```python
from build123d import *

# Parameters (mm, degrees)
F2_R = 5.08


with BuildPart() as f1:
    # F0 (on Right) → F1 (revolve)
    with BuildSketch(Plane.YZ):
        Polygon((-64.897239, 0), (0, 0), (86.770147, 0), (93.20876, 4.190467), (93.20876, 11.651084), (89.325145, 22.790901), (81.864543, 22.790901), (77.878736, 14.819287), (73.484123, 7.767476), (59.891507, 7.767476), (56.518897, 12.67308), (51.000088, 19.827098), (44.970281, 24.630502), (32.7297, 28.463185), (22.135049, 28.463185), (11.288136, 24.301), (4.981786, 17.364018), (0, 9.039648), (-64.897239, 9.039648), align=None)
    revolve(axis=Axis((0, -32.44862, 0), (0, -1, 0)))

    # F2
    f2_edges = [f1.edges().sort_by_distance(p)[0] for p in [
        (0, -64.897239, -9.039648),
    ]]
    fillet(f2_edges, radius=F2_R)


solid = f1.part
```
The model under review builds one solid part; all positions refer to its coordinate system, in mm. A direction names the side the tool comes from. Give positions to 0.01 mm unless a question says otherwise; leave off trailing zeros. Write each loop counter-clockwise with the first axis right and the second up, starting at its lowest first coordinate (ties: lowest second). Pieces come first, ordered by that corner, then holes.
(1) Tool access review of faces 4 (the cylindrical face through (-8.55, 27.36, 27.15)), 5 (the cylindrical face through (13.868, 85.543, -18.086)), 6 (the cylindrical face through (-7.7, 66.59, -1.01)): name each direction out of +Z, -Z, +X, -X, +Y, -Y from which nothing blocks a thin tool from reaching the whole face with its end or side.
(2) Consider section A-A, the plane y = -28.5. Give the boundary of the cut face in (x, z), and give its area (3 significant figures).
(3) For P1, Ø1, axis at y = 33.5, z = -3, coming from the +X side; P2, Ø8, axis at x = 17.5, z = -4, coming from the +Y side; P3, Ø10, axis at x = 0, y = 6, coming from the -Z side, all flat-tipped, find the tip position at first contact; note any pin that passes through.
(4) To check wall thickness, follow L1, parallel to Y at x = -12, z = 10; L2, parallel to Y at x = -4.5, z = -17; L3, parallel to X at y = 37, z = 12. State the ranges of each line that lie inside material, in increasing order.
(5) The part is to be moulded in two halves that separate along Y. For faces 1 (the conical face through (1.47, 89.32, 0.77)), 2 (the cylindrical face through (-2.72, -30.33, 8.62)), 3 (the conical face through (-4.57, 78.07, 14.5)), say which applies: released by +Y, released by -Y, zero draft, split by the parting line, or undercut.
Returned:
1. face 4: +Y, -Y
1. face 5: +Y
1. face 6: none
2. outline: circle Ø18.08 at (0, 0)
2. area: 257 mm2
3. P1: stops at x = 28.23
3. P2: stops at y = 92.41
3. P3: stops at z = -23.98
4. L1: y = 3.94 to 54.25, 78.28 to 91.82
4. L2: y = 5.18 to 52.73, 79.26 to 91.14
4. L3: x = -24.33 to 24.33
5. face 1: released by +Y
5. face 2: zero draft
5. face 3: undercut
